Model file for the job. Use its own axes, mm. Give positions to 0.01 mm unless a question says otherwise; leave off trailing zeros. Write each loop counter-clockwise with the first axis right and the second up, starting at its lowest first coordinate (ties: lowest second). Pieces come first, ordered by that corner, then holes. Notation, with made-up numbers: (15, 10.25) - (47, 10.25) arc R13 ccw to (47, 30.25) - close; hole circle Ø2 at (41, 68.5). An arc over 180 degrees is marked (long way). One line per item, written item: value. Start each with the question number.
(1) Cut at B-B, the plane x = 11. List the corners of the cut face in (y, z), and give its area (3 significant figures).
(2) Mould opens along Y. For faces 1 (the face through (0, 0, 15)), 2 (the face through (-9.74, -14.14, 7.6)), 3 (the face through (0, 30, 7)), 4 (the face through (10.909, 10.435, 7.605)) say: pulls with the +Y half, pulls with the -Y half, needs draft (parallel to the pull), parting line crosses it, or undercut.
(3) Cut at A-A, the plane z = 8.5. List the corners of the cut face in (x, y).
(4) Probe L1, parallel to Y at x = 11, z = 11.5; L2, parallel to X at y = -12.5, z = 4; L3, parallel to Y at x = 0, z = 9.5. List the from-to ranges inside material, lowest first.
(5) Cut at C-C, the plane y = -12.5. List the corners of the cut face in (x, z).
(6) Cut at D-D, the plane y = -20. List the corners of the cut face in (x, z).
Autodesk Inventor part; units mm, degrees
ref_plane "YZ Plane" through (0, 0, 0) normal (1, 0, 0) x (0, 1, 0)
ref_plane "XZ Plane" through (0, 0, 0) normal (0, 1, 0) x (-1, 0, 0)
ref_plane "XY Plane" through (0, 0, 0) normal (0, 0, 1) x (1, 0, 0)
sketch "Skizze1" plane through (0, 0, 0) normal (0, 0, 1) x (1, 0, 0)
  line L0 (-17, 30) -> (17, 30)
  line L1 (17, 30) -> (17, -30)
  line L2 (17, -30) -> (-17, -30)
  line L3 (-17, -30) -> (-17, 30)
  line L4 (-23.8, 0) -> (23.8, 0)
  line L5 (0, -42) -> (0, 42)
  point P0 (0, 0)
  dimension "d0" = 34
  dimension "d1" = 60
extrude "Extrusion1" add sketch "Skizze1" along normal blind 15
sketch "Skizze2" plane through (0, 0, 0) normal (0, 0, -1) x (-1, 0, 0)
  line L0 (23.8, 0) -> (-23.8, 0)
  line L1 (0, -42) -> (0, 42)
  line L2 (11, 12.5) -> (-11, 12.5)
  line L3 (-11, 12.5) -> (-11, -12.5)
  line L4 (-11, -12.5) -> (11, -12.5)
  line L5 (11, -12.5) -> (11, 12.5)
  point P0 (0, 0)
  dimension "d4" = 22
  dimension "d5" = 25
hole "Bohrung1" at (-11, 12.5, 0) at (-11, -12.5, 0) at (11, -12.5, 0) at (11, 12.5, 0) direction (0, 0, 1) diameter 4.134 end through all
sketch "Skizze3" plane through (0, 0, 15) normal (0, 0, 1) x (1, 0, 0)
  circle A0 centre (0, 20) radius 2.75
  circle A1 centre (0, -20) radius 2.75
  point P0 (0, 0)
hole "Bohrung2" at (0, 20, 15) at (0, -20, 15) direction (0, 0, -1) diameter 4.134 end through all
properties part number "1_0204_011"
Answers follow:
1. outline: (-30, 0) - (-14.57, 0) - (-14.57, 15) - (-30, 15) - close; (-10.43, 0) - (10.43, 0) - (10.43, 15) - (-10.43, 15) - close; (14.57, 0) - (30, 0) - (30, 15) - (14.57, 15) - close
1. area: 776 mm²
2. face 1: needs draft
2. face 2: undercut
2. face 3: pulls with the +Y half
2. face 4: undercut
3. outline: (-17, -30) - (17, -30) - (17, 30) - (-17, 30) - close; hole circle Ø4.13 at (-11, -12.5); hole circle Ø4.13 at (-11, 12.5); hole circle Ø4.13 at (0, -20); hole circle Ø4.13 at (0, 20); hole circle Ø4.13 at (11, -12.5); hole circle Ø4.13 at (11, 12.5)
4. L1: y = -30 to -14.57, -10.43 to 10.43, 14.57 to 30
4. L2: x = -17 to -13.07, -8.93 to 8.93, 13.07 to 17
4. L3: y = -30 to -22.07, -17.93 to 17.93, 22.07 to 30
5. outline: (-17, 0) - (-13.07, 0) - (-13.07, 15) - (-17, 15) - close; (-8.93, 0) - (8.93, 0) - (8.93, 15) - (-8.93, 15) - close; (13.07, 0) - (17, 0) - (17, 15) - (13.07, 15) - close
6. outline: (-17, 0) - (-2.07, 0) - (-2.07, 15) - (-17, 15) - close; (2.07, 0) - (17, 0) - (17, 15) - (2.07, 15) - close
